Could you check a few things on this model? Use its own coordinates, in mm. Face numbers are marked on the shaded views. A direction names the side the tool comes from. Give positions to 0.01 mm unless a question says otherwise; leave off trailing zeros. Loops run counter-clockwise (first coordinate to the right, second up) from the corner with the lowest first, then second, coordinate; pieces in that order, holes last. Notation, with made-up numbers: M 29.5,35.25 L 83.5,35.25 A16 cw 83.5,56.25 Z; hole C 65.25,60.25 d1. An arc over 180 degrees is marked long. Use a Markdown table: item, result. Add a question column.
1) Will these pins go through, and if not, where does the flat tip stop? pin 1 Ø9 at (x, y) = (11, -5) entering from +Z; pin 2 Ø8 at (y, z) = (-95, -12) entering from -X; pin 3 Ø8 at (x, y) = (11, -95) entering from -Z.
2) Suppose I cut it at B-B on y = -95. Count the separate pieces of the cut face and the enclosed holes in it, and give its area (3 significant figures).
3) Suppose I cut it at A-A on y = 32.5. List the corners of the cut face in (x, z) for me.
4) Suppose I cut it at D-D on x = 0. List the corners of the cut face in (y, z) for me, and give its area (3 significant figures).
5) Which directions (+Z, -Z, +X, -X, +Y, -Y) give clear straight access to the entire face, cutting with the end or side of a thin tool? Please do the marked faces 1 and 2.
6) If I drill on line 1 along Z through (x, y) = (-6, 69); line 2 along X through (y, z) = (-38.5, -7); line 3 along X through (y, z) = (-95, 0.2), over which ranges is the centre line in solid material (lowest first)? Write a range as [from, to].
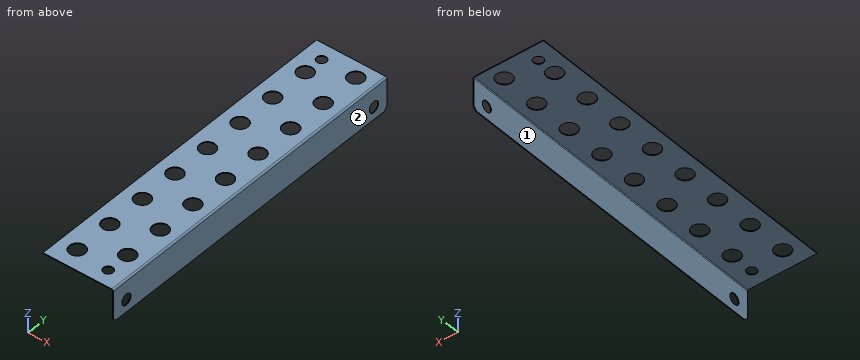
```python
from build123d import *

# Parameters (mm, degrees)
SKETCH2_W                          = 44
SKETCH2_H                          = 210
BOSS_EXTRUDE1_DEPTH                = 0.5
SKETCH3_R                          = 5
CUT_EXTRUDE1_DEPTH                 = 108.281172626
LPATTERN1_COUNT                    = 8
LPATTERN1_PITCH                    = 25
EDGE_FLANGE1_STRIP_W               = 3
EDGE_FLANGE1_STRIP_H               = 0.5
EDGE_FLANGE1_STRIP_CUT_DEPTH       = 210
EDGE_FLANGE1_DEPTH                 = 210
F_7_0_7_DIAMETER_HOLE1_D           = 7
F_7_0_7_DIAMETER_HOLE1_DEPTH       = 60
F_7_0_7_DIAMETER_HOLE1_CSINK_D     = 7.05
F_7_0_7_DIAMETER_HOLE1_CSINK_ANGLE = 90
F_7_0_7_DIAMETER_HOLE1_TIP         = 2.103012167
BREAK_CORNER1_START                = 86.974134086
BREAK_CORNER1_OUTLINE_W            = 3
BREAK_CORNER1_OUTLINE_H            = 149.974134086
BREAK_CORNER1_DEPTH                = 1.414213562
BREAK_CORNER1_START_2              = -61.518289963
BREAK_CORNER1_2_OUTLINE_W          = 3
BREAK_CORNER1_2_OUTLINE_H          = 2.025865914
BREAK_CORNER1_2_DEPTH              = 2.828427125
SKETCH17_R                         = 3.1
CUT_EXTRUDE2_DEPTH                 = 10


# Read off the part's stored shape, not the designer's step: Break-Corner1
# Sheet-metal steps are written as plain solids
with BuildPart() as part:
    # Sketch2 → Boss-Extrude1 (new body)
    with BuildSketch(Plane.XY):
        Rectangle(SKETCH2_W, SKETCH2_H)
    extrude(amount=BOSS_EXTRUDE1_DEPTH)

    # Sketch3 → Cut-Extrude1 (cut, through all)
    with BuildSketch(Plane.XY.offset(0.5)):
        with Locations((11, 95)):
            Circle(SKETCH3_R)
        with Locations((-10.650635095, 82.5)):
            Circle(SKETCH3_R)
    cut_extrude1 = extrude(amount=-CUT_EXTRUDE1_DEPTH, mode=Mode.SUBTRACT)

    # LPattern1: Cut-Extrude1 ×8
    with Locations(*[(0, -i * LPATTERN1_PITCH, 0) for i in range(1, LPATTERN1_COUNT)]):
        add(cut_extrude1, mode=Mode.SUBTRACT)

    # Edge-Flange1 strip (across the edge) → Edge-Flange1 strip cut (cut)
    with BuildSketch(Plane(origin=(22, 105, 0), x_dir=(-1, 0, 0), z_dir=(0, -1, 0))):
        with Locations((-1, -0.25)):
            Rectangle(EDGE_FLANGE1_STRIP_W, EDGE_FLANGE1_STRIP_H)
    extrude(amount=EDGE_FLANGE1_STRIP_CUT_DEPTH, mode=Mode.SUBTRACT)

    # Edge-Flange1 section (across the edge) → Edge-Flange1 (add)
    with BuildSketch(Plane(origin=(22, 105, 0), x_dir=(-1, 0, 0), z_dir=(0, -1, 0))):
        with BuildLine():
            Line((-0.5, 0.5), (-0.5, 20))
            Line((-0.5, 20), (0, 20))
            Line((0, 20), (0, 0.5))
            ThreePointArc((0, 0.5), (0.146446609, 0.146446609), (0.5, 0))
            Line((0.5, 0), (0.5, -0.5))
            ThreePointArc((0.5, -0.5), (-0.207106781, -0.207106781), (-0.5, 0.5))
        make_face()
    extrude(amount=EDGE_FLANGE1_DEPTH)

    # Ø7.0 (7) Diameter Hole1
    with Locations(Plane(origin=(22.5, 0, 0), x_dir=(0, 0, -1), z_dir=(1, 0, 0))):
        with Locations((12, 95), (12, -95)):
            CounterSinkHole(F_7_0_7_DIAMETER_HOLE1_D / 2, F_7_0_7_DIAMETER_HOLE1_CSINK_D / 2, depth=F_7_0_7_DIAMETER_HOLE1_DEPTH, counter_sink_angle=F_7_0_7_DIAMETER_HOLE1_CSINK_ANGLE)
            with Locations((0, 0, -(F_7_0_7_DIAMETER_HOLE1_DEPTH + F_7_0_7_DIAMETER_HOLE1_TIP / 2))):  # 118° drill point
                Cone(0, F_7_0_7_DIAMETER_HOLE1_D / 2, F_7_0_7_DIAMETER_HOLE1_TIP, mode=Mode.SUBTRACT)

    # Break-Corner1 outline → Break-Corner1 (cut)
    with BuildSketch(Plane(origin=(0, 0, 0), x_dir=(1, 0, 0), z_dir=(0, 0.707106781186545, -0.70710678118655)).offset(BREAK_CORNER1_START)):
        with Locations((22.5, 11.987067043)):
            Rectangle(BREAK_CORNER1_OUTLINE_W, BREAK_CORNER1_OUTLINE_H)
    extrude(amount=BREAK_CORNER1_DEPTH, mode=Mode.SUBTRACT)

    # Break-Corner1 2 outline → Break-Corner1 2 (cut)
    with BuildSketch(Plane(origin=(0, 0, 0), x_dir=(1, 0, 0), z_dir=(0, 0.707106781186545, -0.70710678118655)).offset(BREAK_CORNER1_START_2)):
        with Locations((22.5, 87.987067043)):
            Rectangle(BREAK_CORNER1_2_OUTLINE_W, BREAK_CORNER1_2_OUTLINE_H)
    extrude(amount=BREAK_CORNER1_2_DEPTH, mode=Mode.SUBTRACT)

    # Sketch17 → Cut-Extrude2 (cut)
    with BuildSketch(Plane.XY):
        with Locations((-10.650635095, 95)):
            Circle(SKETCH17_R)
        with Locations((11, -95)):
            Circle(SKETCH17_R)
    extrude(amount=CUT_EXTRUDE2_DEPTH, mode=Mode.SUBTRACT)


solid = part.part
```
Answer block:
| question | item | result |
|---|---|---|
| 1 | pin 1 | passes through |
| 1 | pin 2 | stops at x = 22 |
| 1 | pin 3 | stops at z = 0 |
| 2 | separate pieces | 4 |
| 2 | enclosed holes | 0 |
| 2 | area | 21.2 mm^2 |
| 3 | outline | M -22,0 L -15.65,0 L -15.65,0.5 L -22,0.5 Z; M -5.65,0 L 21.5,0 A0.5 cw 22,-0.5 L 22,-20 L 22.5,-20 L 22.5,-0.5 A1 ccw 21.5,0.5 L -5.65,0.5 Z |
| 4 | outline | M -105,0 L 105,0 L 105,0.5 L -105,0.5 Z |
| 4 | area | 105 mm^2 |
| 5 | face 1 | -Z, -X, +Y, -Y |
| 5 | face 2 | +Z, -Z, +X, +Y, -Y |
| 6 | line 1 | z = [0, 0.5] |
| 6 | line 2 | x = [22, 22.5] |
| 6 | line 3 | x = [-22, -14.98], [-6.32, 7.9], [14.1, 22.21] |
